Design review of the part shown in the three views and the two pictorial views. Dimensions are in mm from the part's minimum x, y and z. A direction names the side the tool comes from. Give positions to 0.01 mm unless a question says otherwise; leave off trailing zeros. Write each loop counter-clockwise with the first axis right and the second up, starting at its lowest first coordinate (ties: lowest second). Pieces come first, ordered by that corner, then holes. Notation, with made-up numbers: M 38,-14.5 L 94,-14.5 A16 cw 94,5.5 Z; hole C 61,27.25 d1. An arc over 180 degrees is marked long. Use one line per item in the form item = value. Start each with the question number.
Q1. Tool access review of the marked faces 5 and 6: name each direction out of +Z, -Z, +X, -X, +Y, -Y from which nothing blocks a thin tool from reaching the whole face with its end or side.
Q2. Consider section A-A on x = 4. Write out the cut boundary in (y, z).
Q3. Consider section C-C on z = 6. Write out the cut boundary in (x, y) (3 decimals).
Q4. Consider section D-D on z = 1.25. Write out the cut boundary in (x, y), and give its area (3 significant figures).
Q5. Consider section B-B on y = 9.5. Write out the cut boundary in (x, z).
Q6. Mouldability with a two-part tool opening along Z and no side actions: class the marked faces 1, 2, 3 and 4 as released by +Z, released by -Z, zero draft, split by the parting line, or undercut.
Q7. Clearance check with flat-ended pins moving along their axes: pin 1 Ø0.5 at (y, z) = (14, 0.5) entering from +X; pin 2 Ø1.4 at (x, z) = (4.5, 0.5) entering from +Y; pin 3 Ø4 at (x, y) = (1.5, 7) entering from -Z. State where each tip first meets the part, or that it passes through.
Q8. For probe 1 along X at (y, z) = (6.5, 5.8); probe 2 along Z at (x, y) = (5, 7.5); probe 3 along X at (y, z) = (7.25, 6.75), list the stretches that pass through material, from the lowest coordinate up. Write a range as [from, to].
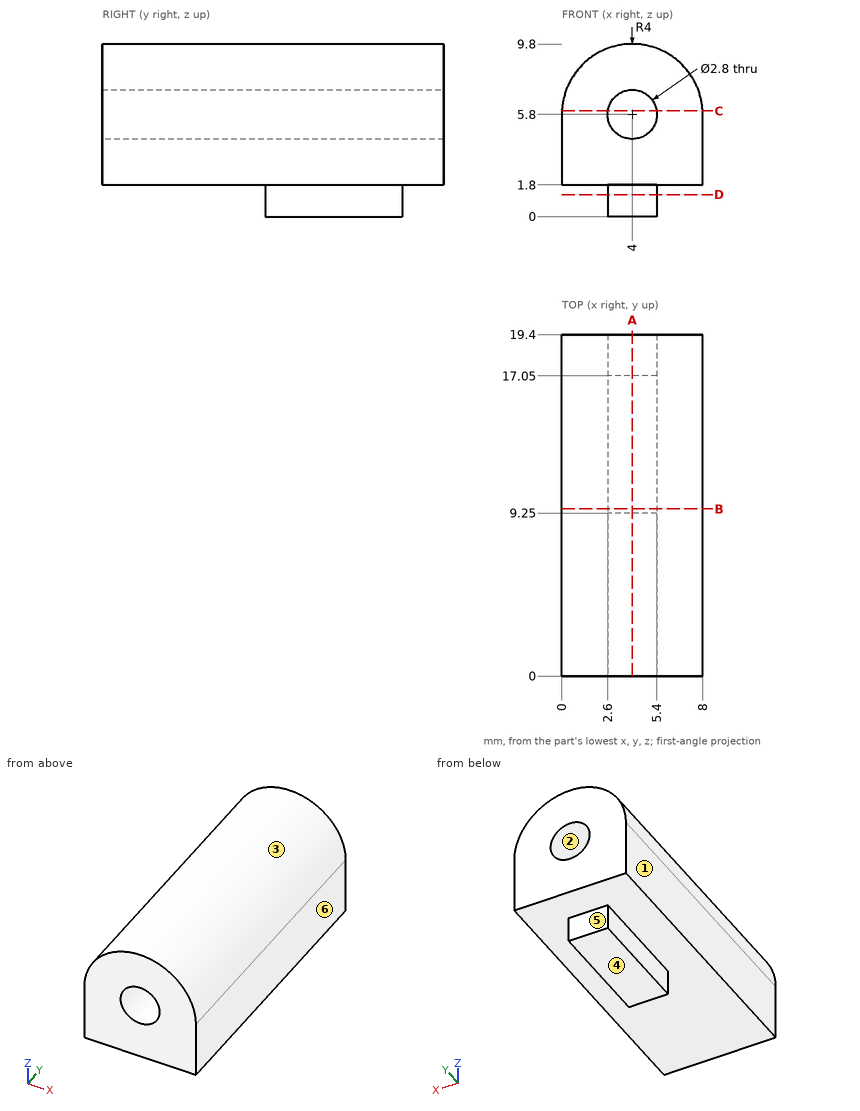
Working result:
q1.face_5 = -Z, +X, -X, +Y
q1.face_6 = +Z, -Z, +X, +Y, -Y
q2.outline = M 0,1.8 L 9.25,1.8 L 9.25,0 L 17.05,0 L 17.05,1.8 L 19.4,1.8 L 19.4,4.4 L 0,4.4 Z; M 0,7.2 L 19.4,7.2 L 19.4,9.8 L 0,9.8 Z
q3.outline = M 0.005,0 L 2.614,0 L 2.614,19.4 L 0.005,19.4 Z; M 5.386,0 L 7.995,0 L 7.995,19.4 L 5.386,19.4 Z
q4.outline = M 2.6,9.25 L 5.4,9.25 L 5.4,17.05 L 2.6,17.05 Z
q4.area = 21.8 mm²
q5.outline = M 0,1.8 L 2.6,1.8 L 2.6,0 L 5.4,0 L 5.4,1.8 L 8,1.8 L 8,5.8 A4 ccw 0,5.8 Z; hole C 4,5.8 d2.8
q6.face_1 = zero draft
q6.face_2 = undercut
q6.face_3 = released by +Z
q6.face_4 = released by -Z
q7.pin_1 = 5.4
q7.pin_2 = 17.05
q7.pin_3 = 1.8
q8.probe_1 = [0, 2.6], [5.4, 8]
q8.probe_2 = [1.8, 4.82], [6.78, 9.67]
q8.probe_3 = [0.11, 2.97], [5.03, 7.89]
